The drawing under review shows one solid part. Ordinate dimensions are in mm from its lowest x, y, z. Round coordinates to 2 decimals unless told otherwise and drop trailing zeros. Order: outer loops, then holes, each group sorted by start corner. A loop starts at its lowest first (then second) coordinate and runs counter-clockwise, first axis right, second up. Notation, with made-up numbers: (78, -20) -> (120, -20) arc R29 ccw to (120, 1) -> close; hole circle Ø4 at (9.25, 48.5). An arc over 180 degrees is marked (long way). Use a Markdown table: item, result. Add a question column.
1) Wall thickness on line 1 along Y through (x, z) = (5, 1); line 2 along X through (y, z) = (85, 1.4); line 3 along Y through (x, z) = (74, 4.9): over which ranges is each line inside the solid? List them lowest first. Write a range as [from, to].
2) Clearance check with flat-ended pins moving along their axes: P1, Ø6, axis at x = 119.5, y = 43.5, coming from the +Z side; P2, Ø8, axis at x = 26.5, y = 13.5, coming from the +Z side. State where each tip first meets the part, or that it passes through.
3) Consider section C-C (z = 4.95). State the section outline as (x, y) points, plus the area to 3 significant figures.
4) Consider section A-A (y = 39). State the section outline as (x, z) points.
5) Consider section B-B (x = 51.5). State the section outline as (y, z) points, plus the area to 3 significant figures.
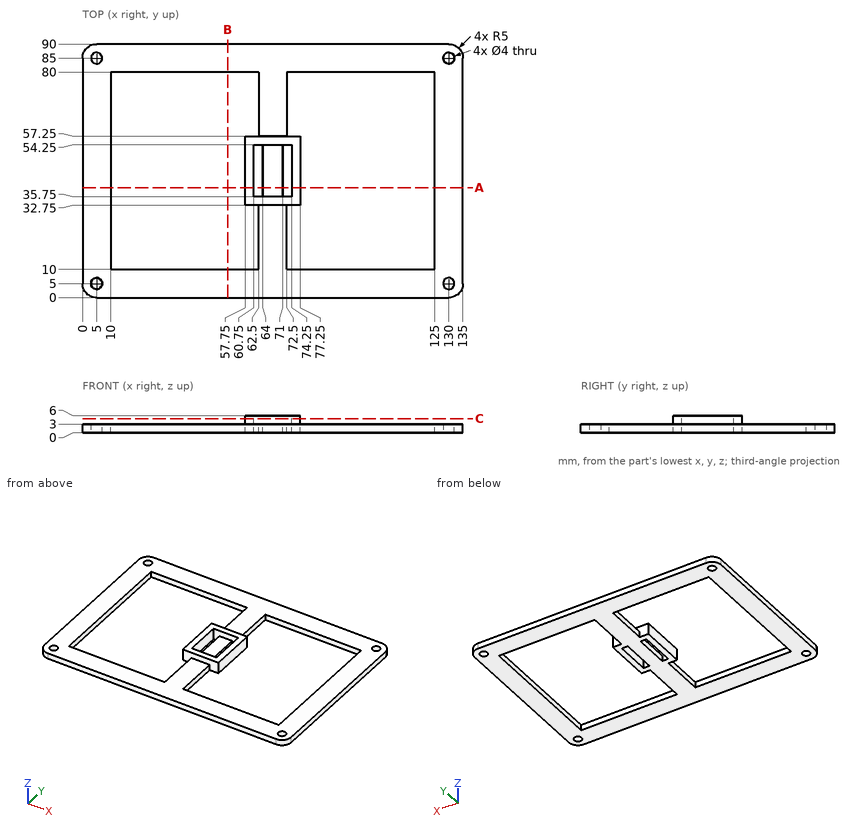
Results list:
| question | item | result |
|---|---|---|
| 1 | line 1 | [0, 3], [7, 83], [87, 90] |
| 1 | line 2 | [0, 3], [7, 128], [132, 135] |
| 1 | line 3 | [32.75, 35.75], [54.25, 57.25] |
| 2 | P1 | through |
| 2 | P2 | z = 3 |
| 3 | outline | (57.75, 32.75) -> (77.25, 32.75) -> (77.25, 57.25) -> (57.75, 57.25) -> close; hole (60.75, 35.75) -> (74.25, 35.75) -> (74.25, 54.25) -> (60.75, 54.25) -> close |
| 3 | area | 228 mm2 |
| 4 | outline | (0, 0) -> (10, 0) -> (10, 3) -> (0, 3) -> close; (57.75, 0) -> (60.75, 0) -> (60.75, 6) -> (57.75, 6) -> close; (64, 0) -> (71, 0) -> (71, 3) -> (64, 3) -> close; (74.25, 0) -> (77.25, 0) -> (77.25, 6) -> (74.25, 6) -> close; (125, 0) -> (135, 0) -> (135, 3) -> (125, 3) -> close |
| 5 | outline | (0, 0) -> (10, 0) -> (10, 3) -> (0, 3) -> close; (80, 0) -> (90, 0) -> (90, 3) -> (80, 3) -> close |
| 5 | area | 60.0 mm2 |
